```python
from build123d import *

# Parameters (mm, degrees)
F1_DEPTH = 127


with BuildPart() as f1:
    # F0 (on Front) → F1 (new body)
    with BuildSketch(Plane.XZ):
        with BuildLine():
            Line((-563.192896, -166.407167), (-449.012806, -449.012806))
            Line((-449.012806, -449.012806), (-166.407167, -563.192896))
            Line((-166.407167, -563.192896), (57.539014, -254.957421))
            ThreePointArc((57.539014, -254.957421), (102.32825, -117.110326), (147.117486, -254.957421))
            Line((147.117486, -254.957421), (371.063668, -563.192896))
            Line((371.063668, -563.192896), (653.669306, -449.012806))
            Line((653.669306, -449.012806), (767.849396, -166.407167))
            Line((767.849396, -166.407167), (459.613921, 57.539014))
            ThreePointArc((459.613921, 57.539014), (321.766826, 102.32825), (459.613921, 147.117486))
            Line((459.613921, 147.117486), (767.849396, 371.063668))
            Line((767.849396, 371.063668), (653.669306, 653.669306))
            Line((653.669306, 653.669306), (371.063668, 767.849396))
            Line((371.063668, 767.849396), (147.117486, 459.613921))
            ThreePointArc((147.117486, 459.613921), (102.32825, 321.766826), (57.539014, 459.613921))
            Line((57.539014, 459.613921), (-166.407167, 767.849396))
            Line((-166.407167, 767.849396), (-449.012806, 653.669306))
            Line((-449.012806, 653.669306), (-563.192896, 371.063668))
            Line((-563.192896, 371.063668), (-254.957421, 147.117486))
            ThreePointArc((-254.957421, 147.117486), (-117.110326, 102.32825), (-254.957421, 57.539014))
            Line((-254.957421, 57.539014), (-563.192896, -166.407167))
        make_face()
    extrude(amount=F1_DEPTH)


solid = f1.part
```
Model file for the job. Use its own axes, mm. A direction names the side the tool comes from. Give positions to 0.01 mm unless a question says otherwise; leave off trailing zeros. Loops run counter-clockwise (first coordinate to the right, second up) from the corner with the lowest first, then second, coordinate; pieces in that order, holes last. Notation, with made-up numbers: (34.25, 87.5) - (41.25, 87.5) arc R18 ccw to (41.25, 109.5) - close; hole circle Ø10 at (84, 72.25). An arc over 180 degrees is marked (long way). One line per item, written item: value. Start each with the question number.
1. Pin check, flat tips, straight feed: pin 1 (8 mm diameter, centred on x = 562, y = -82, fed in from +Z); pin 2 (3 mm diameter, centred on x = -265, y = -73.5, fed in from +Z); pin 3 (5 mm diameter, centred on x = -380, y = -100, fed in from -Z). Stop position of each tip, or through.
2. Slice it at A-A (y = -21). List the corners of the cut face in (x, z), plus the area to 3 significant figures.
3. Slice it at B-B (z = -477). List the corners of the cut face in (x, y).
4. Slice it at D-D (z = 391). List the corners of the cut face in (x, y), plus the area to 3 significant figures.
5. Which spindle directions (+Z, -Z, +X, -X, +Y, -Y) get a long thin tool onto all of the face, cutting with end or side? Do faces 1 (the flat face through (-411.233, -62.611, 260.658)), 2 (the flat face through (615.89, -62.61, -56)), 3 (the flat face through (-52.866, -62.611, 611.574)). Say none if no direction does.
6. Pull direction X, two halves, no side cores. Call faces 4 (the flat face through (611.57, -62.61, 257.52)), 5 (the flat face through (93, 0, 112)), 6 (the flat face through (-56, -62.61, -411.23)), 7 (the flat face through (-505.304, -62.611, 514.345)): pulls with the +X half, pulls with the -X half, needs draft (parallel to the pull), parting line crosses it, or undercut.
7. Slice it at C-C (x = -31). List the corners of the cut face in (y, z), plus the area to 3 significant figures.
8. Probe L1, parallel to Z at x = 165.5, y = -41; L2, parallel to Z at x = -427.5, y = -15; L3, parallel to X at y = -47.5, z = -229. List the from-to ranges inside material, lowest first. Write a range as from..to.
Solution:
1. pin 1: stops at z = 692.32
1. pin 2: stops at z = 728.62
1. pin 3: stops at z = -477.91
2. outline: (-563.19, -166.41) - (-449.01, -449.01) - (-166.41, -563.19) - (57.54, -254.96) arc R76.2 cw (long way) to (147.12, -254.96) - (371.06, -563.19) - (653.67, -449.01) - (767.85, -166.41) - (459.61, 57.54) arc R76.2 cw (long way) to (459.61, 147.12) - (767.85, 371.06) - (653.67, 653.67) - (371.06, 767.85) - (147.12, 459.61) arc R76.2 cw (long way) to (57.54, 459.61) - (-166.41, 767.85) - (-449.01, 653.67) - (-563.19, 371.06) - (-254.96, 147.12) arc R76.2 cw (long way) to (-254.96, 57.54) - close
2. area: 1,130,000 mm^2
3. outline: (-379.74, -127) - (-103.78, -127) - (-103.78, 0) - (-379.74, 0) - close; (308.44, -127) - (584.4, -127) - (584.4, 0) - (308.44, 0) - close
4. outline: (-555.14, -127) - (26.45, -127) - (26.45, 0) - (-555.14, 0) - close; (178.21, -127) - (759.79, -127) - (759.79, 0) - (178.21, 0) - close
4. area: 148,000 mm^2
5. face 1: -X, +Y, -Y
5. face 2: +X, +Y, -Y
5. face 3: +Z, +Y, -Y
6. face 4: pulls with the +X half
6. face 5: needs draft
6. face 6: undercut
6. face 7: pulls with the -X half
7. outline: (-127, -376.82) - (0, -376.82) - (0, 581.48) - (-127, 581.48) - close
7. area: 122,000 mm^2
8. L1: z = -280.26..-235.92, -150.7..355.35, 440.58..484.92
8. L2: z = -457.7..-67.82, 272.48..662.36
8. L3: x = -537.9..35, 169.65..742.56
